Geometry check sheet. Reference: the model listing, model coordinates, mm. Face numbers are marked on the shaded views. Round coordinates to 2 decimals unless told otherwise and drop trailing zeros. Loops run counter-clockwise (first coordinate to the right, second up) from the corner with the lowest first, then second, coordinate; pieces in that order, holes last.
```python
from build123d import *

# Parameters (mm, degrees)
FILLET1_R          = 2
SKETCH3_R          = 1.15
CUT_EXTRUDE1_DEPTH = 10
CIRPATTERN1_COUNT  = 4


with BuildPart() as part:
    # Sketch2 → Revolve1 (revolve)
    with BuildSketch(Plane.XY, mode=Mode.PRIVATE) as revolve1_sk:
        Polygon((-31, 0), (-31, 10), (-15.639434665, 25.360565335), (-19.639434665, 25.360565335), (-35, 10), (-35, 0), align=None)
    revolve(revolve1_sk.sketch.rotate(Axis((0, 0, 0), (0, 1, 0)), 180), axis=Axis((0, 0, 0), (0, 1, 0)))

    # Fillet1
    # the kernel refuses this fillet: 2 mm, written as the material it takes off along each edge
    with BuildSketch(Plane(origin=(0, 25.360565335, 0), x_dir=(1, 0, 0), z_dir=(0, 0, 1))) as fillet1_piece_1:
        with BuildLine():
            CenterArc((20.340836733, -1.872974943), FILLET1_R, 110.530199479, 114.469800521)
            Line((19.639434665, 0), (19.625406624, 0.037459499))
            ThreePointArc((19.625406624, 0.037459499), (17.639434665, 0.04), (15.639434665, 0.04))
            Line((15.639434665, 0.04), (15.611150394, -0.028284271))
            Line((15.611150394, -0.028284271), (18.8983389, -3.315472777))
            Line((18.8983389, -3.315472777), (18.926623171, -3.287188506))
        make_face()
    revolve(axis=Axis((0, 25.360565335, 0), (0, 1, 0)), mode=Mode.SUBTRACT)

    # Sketch3 → Cut-Extrude1 (cut)
    with BuildSketch(Plane.XZ):
        with Locations(Location((0, 33, 0), (0, 0, 270))):
            Circle(SKETCH3_R)
    cut_extrude1 = extrude(amount=-CUT_EXTRUDE1_DEPTH, mode=Mode.SUBTRACT)

    # CirPattern1: Cut-Extrude1 ×4 about axis
    cirpattern1_axis = Axis((0, 0, 0), (0, 1, 0))
    for i in range(1, CIRPATTERN1_COUNT):
        add(cut_extrude1.rotate(cirpattern1_axis, i * 360 / CIRPATTERN1_COUNT), mode=Mode.SUBTRACT)


solid = part.part
```
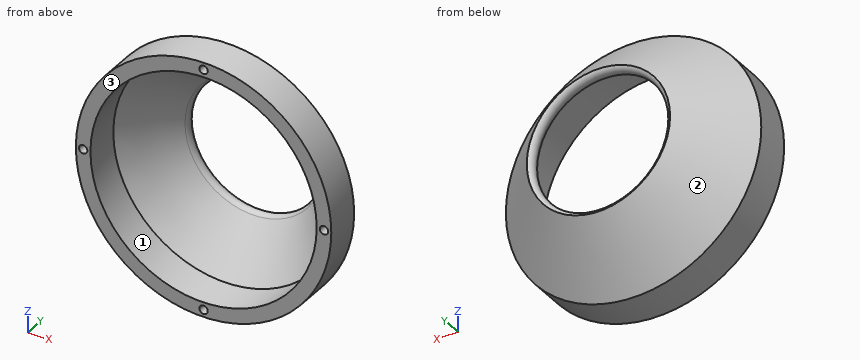
1) Gauge pin test, flat ends, axial feed: pin 1 (2 mm diameter, centred on y = 4.5, z = -3.5, fed in from +X); pin 2 (1.5 mm diameter, centred on x = -13.5, y = 6.5, fed in from -Z); pin 3 (0.7 mm diameter, centred on x = 0.5, z = 32.5, fed in from -Y). Record the tip position at first contact, or that the pin passes through.
Report:
pin 1: stops at x = 34.91
pin 2: stops at z = -32.6
pin 3: stops at y = 10
2) Sectioned sample at B-B, the plane x = 0. Record the cut outline in (y, z).
Report:
outline: (0, -35) - (10, -35) - (25.36, -19.64) arc R2 ccw to (22.07, -18.93) - (10, -31) - (0, -31) - (0, -31.85) - (10, -31.85) - (10, -34.15) - (0, -34.15) - close; (0, 31) - (10, 31) - (22.07, 18.93) arc R2 ccw to (25.36, 19.64) - (10, 35) - (0, 35) - (0, 34.15) - (10, 34.15) - (10, 31.85) - (0, 31.85) - close
3) Mould release check, pull along X, two halves, no side actions. Record for the marked faces 1, 2 and 3: +X half, -X half, draft (parallel to the pull), parting line (faces both ways), or undercut.
Report:
face 1: undercut
face 2: parting line
face 3: draft
4) Sectioned sample at D-D, the plane y = 12.75. Record the cut outline in (x, z), then the cut area to 3 significant figures.
Report:
outline: circle Ø64.5 at (0, 0); hole circle Ø56.5 at (0, 0)
area: 760 mm2
5) Scan lines: line 1 along Z through (x, y) = (-22, 2.5); line 2 along X through (y, z) = (2.25, -20.5); line 3 along Z through (x, y) = (2, 4.5). Record each from-to range of solid material in increasing order.
Report:
line 1: z = -27.22 to -21.84, 21.84 to 27.22
line 2: x = -28.37 to -23.25, 23.25 to 28.37
line 3: z = -34.94 to -30.94, 30.94 to 34.94
6) Sectioned sample at C-C, the plane z = 0. Record the cut outline in (x, y).
Report:
outline: (-35, 0) - (-34.15, 0) - (-34.15, 10) - (-31.85, 10) - (-31.85, 0) - (-31, 0) - (-31, 10) - (-18.93, 22.07) arc R2 ccw to (-19.64, 25.36) - (-35, 10) - close; (18.93, 22.07) - (31, 10) - (31, 0) - (31.85, 0) - (31.85, 10) - (34.15, 10) - (34.15, 0) - (35, 0) - (35, 10) - (19.64, 25.36) arc R2 ccw to start
7) Sectioned sample at A-A, the plane y = 7.5. Record the cut outline in (x, z).
Report:
outline: circle Ø70 at (0, 0); hole circle Ø2.3 at (-33, 0); hole circle Ø62 at (0, 0); hole circle Ø2.3 at (0, -33); hole circle Ø2.3 at (0, 33); hole circle Ø2.3 at (33, 0)
